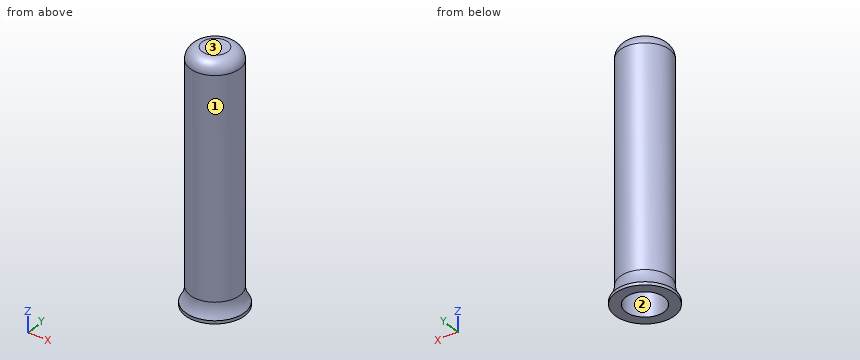
from build123d import *

# Parameters (mm, degrees)
F0_R      = 6.3625068229
F1_DEPTH  = 63.5
F2_R      = 4.7646286231
F3_DEPTH  = 25.146
F4_R      = 7.5920691382
F5_DEPTH  = 0.7874
F6_R      = 4.746247259
F7_DEPTH  = 35.306
F8_R      = 3.0660512242
F10_R     = 4.926173209
F11_DEPTH = 57.658


# Not quite as in the source:
# - a fillet or chamfer that OpenCascade refuses, or shapes differently, is made with other operations: its cross-section is extruded or revolved along the edge and cut away or added


with BuildPart() as f1:
    # F0 (on Top) → F1 (new body)
    with BuildSketch(Plane.XY):
        Circle(F0_R)
    extrude(amount=F1_DEPTH)

    # F2 (on face) → F3 (cut)
    with BuildSketch(Plane(origin=(0, 0, 0), x_dir=(1, 0, 0), z_dir=(0, 0, -1))):
        Circle(F2_R)
    extrude(amount=-F3_DEPTH, mode=Mode.SUBTRACT)

    # F4 (on Top) → F5 (join)
    with BuildSketch(Plane.XY):
        Circle(F4_R)
    extrude(amount=F5_DEPTH)

    # F6 (on face) → F7 (cut)
    with BuildSketch(Plane(origin=(0, 0, 0), x_dir=(1, 0, 0), z_dir=(0, 0, -1))):
        Circle(F6_R)
    extrude(amount=-F7_DEPTH, mode=Mode.SUBTRACT)

    # F8
    f8_edges = [f1.edges().sort_by_distance(p)[0] for p in [
        (-6.362507, 0, 63.5),
    ]]
    fillet(f8_edges, radius=F8_R)

    # F9: fillet of radius 6.4387075708 on 1 edges, made by hand

    # F9_s1 → F9_t2 (revolve)
    with BuildSketch(Plane.XZ):
        with BuildLine():
            ThreePointArc((6.3625068229, 4.5718102432), (6.6776076879, 2.5822384064), (7.5920691382, 0.7874))
            Line((7.5920691382, 0.7874), (6.3625068229, 0.7874))
            Line((6.3625068229, 0.7874), (6.3625068229, 4.5718102432))
        make_face()
    revolve(axis=Axis((0, 0, 0.7874), (0, 0, -1)))

    # F10 (on Top) → F11 (cut)
    with BuildSketch(Plane.XY):
        Circle(F10_R)
    extrude(amount=F11_DEPTH, mode=Mode.SUBTRACT)


solid = f1.part
Geometry check sheet. Reference: the model listing, model coordinates, mm. Face numbers are marked on the shaded views. Give positions to 0.01 mm unless a question says otherwise; leave off trailing zeros. Order: outer loops, then holes, each group sorted by start corner. A loop starts at its lowest first (then second) coordinate and runs counter-clockwise, first axis right, second up. Notation, with made-up numbers: M -35.75,-4.75 L 1.25,-4.75 A25 cw 1.25,14.25 Z; hole C -38.75,70 d4. An arc over 180 degrees is marked long. Use a Markdown table: item, result.
Item 1: Section check A-A (y = 0). Record the cut outline in (x, z), and give its area (3 significant figures).
Answers follow:
| item | result |
|---|---|
| outline | M -7.59,0 L -4.93,0 L -4.93,57.66 L 4.93,57.66 L 4.93,0 L 7.59,0 L 7.59,0.79 A6.44 cw 6.36,4.57 L 6.36,60.43 A3.07 ccw 3.3,63.5 L -3.3,63.5 A3.07 ccw -6.36,60.43 L -6.36,4.57 A6.44 cw -7.59,0.79 Z |
| area | 241 mm2 |
Item 2: Draft check along Y on the marked faces 1, 2 and 3. Enter one of: +Y half, -Y half, draft (parallel to the pull), parting line (faces both ways), or undercut.
Answers follow:
| item | result |
|---|---|
| face 1 | parting line |
| face 2 | undercut |
| face 3 | draft |
Item 3: Depth check by flat-ended pin: P1, Ø5, axis at x = 0, y = 2, coming from the -Z side; P2, Ø1.5, axis at y = -4.5, z = 46.5, coming from the -X side; P3, Ø4, axis at y = -4.5, z = 15, coming from the -X side. Enter the tip coordinate at first touch or a pass-through.
Answers follow:
| item | result |
|---|---|
| P1 | stops at z = 57.66 |
| P2 | stops at x = -5.14 |
| P3 | stops at x = -5.85 |
Item 4: Section check C-C (z = 14.5). Record the cut outline in (x, y), and give its area (3 significant figures).
Answers follow:
| item | result |
|---|---|
| outline | C 0,0 d12.73; hole C 0,0 d9.85 |
| area | 50.9 mm2 |
Item 5: Material ranges on line 1 along Y through (x, z) = (0, 43.5); line 2 along X through (y, z) = (3.25, 29); line 3 along X through (y, z) = (-3.5, 5), recorded low to high.
Answers follow:
| item | result |
|---|---|
| line 1 | y = -6.36 to -4.93, 4.93 to 6.36 |
| line 2 | x = -5.47 to -3.7, 3.7 to 5.47 |
| line 3 | x = -5.31 to -3.47, 3.47 to 5.31 |
